```python
from build123d import *

# Parameters (mm, degrees)
BOSS_EXTRUDE1_DEPTH                        = 7
CUT_EXTRUDE1_REACH                         = 39.696
SKETCH2_R                                  = 4
DIAMETER_HOLE1_D                           = 5.5
CBORE_START                                = 4.5
CBORE_FOR_SOCKET_HEAD_CAP_SCREW1_OUTLINE_R = 4
CBORE_FOR_SOCKET_HEAD_CAP_SCREW1_DEPTH     = 4.5
CBORE_FOR_SOCKET_HEAD_CAP_SCREW1_2_OUTLI_R = 2.25
CBORE_FOR_SOCKET_HEAD_CAP_SCREW1_2_DEPTH   = 4.5
TAPPED_HOLE1_D                             = 3.3
CUT_EXTRUDE2_REACH                         = 39.696
SKETCH9_W                                  = 2
SKETCH9_H                                  = 13
SKETCH10_W                                 = 14
SKETCH10_H                                 = 8
CUT_EXTRUDE3_DEPTH                         = 0.4
FILLET1_R                                  = 1
CHAMFER1_SIZE                              = 1


# Read off the part's stored shape, not the designer's step: CBORE for Socket Head Cap Screw1
with BuildPart() as part:
    # Sketch1 → Boss-Extrude1 (new, symmetric)
    with BuildSketch(Plane.XY):
        Polygon((-21, 0), (21, 0), (21, 6), (9, 6), (9, 28), (-9, 28), (-9, 6), (-21, 6), align=None)
    extrude(amount=BOSS_EXTRUDE1_DEPTH, both=True)

    # Sketch2 → Cut-Extrude1 (cut, up to next)
    with BuildSketch(Plane.XY.offset(7), mode=Mode.PRIVATE) as cut_extrude1_sk1:
        with Locations((0, 15)):
            Circle(SKETCH2_R)
    cut_extrude1_tool1 = extrude(cut_extrude1_sk1.sketch, amount=-CUT_EXTRUDE1_REACH, mode=Mode.PRIVATE) & part.part
    add(cut_extrude1_tool1.solids().sort_by_distance((0, 15, 7))[0], mode=Mode.SUBTRACT)

    # Diameter Hole1 (through all)
    with Locations(Plane(origin=(0, 6, 0), x_dir=(1, 0, 0), z_dir=(0, 1, 0))):
        with Locations((-16, 0), (16, 0)):
            Hole(DIAMETER_HOLE1_D / 2)

    # CBORE for Socket Head Cap Screw1 outline → CBORE for Socket Head Cap Screw1 (cut)
    with BuildSketch(Plane.YZ.offset(CBORE_START)):
        with Locations((22.8, 0)):
            Circle(CBORE_FOR_SOCKET_HEAD_CAP_SCREW1_OUTLINE_R)
    extrude(amount=CBORE_FOR_SOCKET_HEAD_CAP_SCREW1_DEPTH, mode=Mode.SUBTRACT)

    # CBORE for Socket Head Cap Screw1 2 outli → CBORE for Socket Head Cap Screw1 2 (cut)
    with BuildSketch(Plane.YZ):
        with Locations((22.8, 0)):
            Circle(CBORE_FOR_SOCKET_HEAD_CAP_SCREW1_2_OUTLI_R)
    extrude(amount=CBORE_FOR_SOCKET_HEAD_CAP_SCREW1_2_DEPTH, mode=Mode.SUBTRACT)

    # Tapped Hole1 (through all)
    with Locations(Plane(origin=(-9, -2.558166827, -1.433608379), x_dir=(0, 0, -1), z_dir=(-1, 0, 0))):
        with Locations((-1.433608379, -25.358166827)):
            Hole(TAPPED_HOLE1_D / 2)

    # Sketch9 → Cut-Extrude2 (cut, up to next)
    with BuildSketch(Plane.XY.offset(7), mode=Mode.PRIVATE) as cut_extrude2_sk1:
        with Locations((0, 21.5)):
            Rectangle(SKETCH9_W, SKETCH9_H)
    cut_extrude2_tool1 = extrude(cut_extrude2_sk1.sketch, amount=-CUT_EXTRUDE2_REACH, mode=Mode.PRIVATE) & part.part
    add(cut_extrude2_tool1.solids().sort_by_distance((0, 21.5, 7))[0], mode=Mode.SUBTRACT)

    # Sketch10 → Cut-Extrude3 (cut)
    with BuildSketch(Plane.XY.offset(7)):
        with Locations((0, 6)):
            Rectangle(SKETCH10_W, SKETCH10_H)
    extrude(amount=-CUT_EXTRUDE3_DEPTH, mode=Mode.SUBTRACT)

    # Fillet1
    fillet1_edges = [part.edges().sort_by_distance(p)[0] for p in [
        (21, 3, 7),
        (-21, 3, -7),
        (15, 6, 7),
        (-21, 6, 0),
        (-9, 6, 0),
        (-9, 28, 0),
        (9, 28, 0),
        (9, 6, 0),
        (21, 6, 0),
        (9, 17, 7),
        (5, 28, 7),
        (-9, 17, 7),
        (-15, 6, 7),
        (-21, 3, 7),
        (-5, 28, -7),
        (-5, 28, 7),
        (-15, 6, -7),
        (-9, 17, -7),
        (5, 28, -7),
        (9, 17, -7),
        (15, 6, -7),
        (21, 3, -7),
    ]]
    fillet(fillet1_edges, radius=FILLET1_R)

    # Chamfer1
    chamfer1_edges = [part.edges().sort_by_distance(p)[0] for p in [
        (0, 11, 7),
        (0, 11, -7),
    ]]
    chamfer(chamfer1_edges, length=CHAMFER1_SIZE - 0.0001)  # a hair under: the kernel refuses the full size


solid = part.part
```
Geometry check sheet. Reference: the model listing, model coordinates, mm. A direction names the side the tool comes from. Round coordinates to 2 decimals unless told otherwise and drop trailing zeros. Order: outer loops, then holes, each group sorted by start corner. A loop starts at its lowest first (then second) coordinate and runs counter-clockwise, first axis right, second up. Notation, with made-up numbers: (80.25, -28) - (113.25, -28) arc R18 ccw to (113.25, -17) - close; hole circle Ø7 at (86.25, 75.5). An arc over 180 degrees is marked (long way). Use a Markdown table: item, result. Add a question column.
1) Section check C-C (y = 15). Record the cut outline in (x, z), then the cut area to 3 significant figures.
2) Thickness scan on line 1 along Z through (x, y) = (3.1, 22.8); line 2 along Z through (x, y) = (-5.5, 22.8); line 3 along X through (y, z) = (26.25, 3). Record the ranges inside material, lowest first.
3) Section check D-D (x = -15.5). Record the cut outline in (y, z), then the cut area to 3 significant figures.
4) Set-up check for faces 4 (the flat face through (13, 6, 0)), 5 (the cylindrical face through (14.93, 5.699, 6.715)), 6 (the cylindrical face through (-8.699, 16.86, 6.715)), 7 (the cylindrical face through (2.726, 20.552, 0.099)), 8 (the conical face through (-0.171, 10.844, -6.16)): record each of +Z, -Z, +X, -X, +Y, -Y from which the full face is reachable in a straight line by a thin tool's end or side.
5) Mould release check, pull along Y, two halves, no side actions. Record for faces 1 (the cylindrical face through (6.719, 26.495, -1.532)), 2 (the cylindrical face through (8.715, 27.699, 0.084)), 3 (the cylindrical face through (-20.715, 2.465, 6.699)): released by +Y, released by -Y, zero draft, split by the parting line, or undercut.
6) Section check A-A (y = 22.8). Record the cut outline in (x, z), then the cut area to 3 significant figures.
7) Gauge pin test, flat ends, axial feed: P1, Ø7, axis at x = 0, y = 15, coming from the +Z side; P2, Ø6, axis at y = 13.5, z = -1.5, coming from the -X side; P3, Ø3, axis at x = 14, z = -1.5, coming from the +Y side; P4, Ø3.5, axis at y = 12.5, z = -2.5, coming from the +X side. Record the tip position at first contact, or that the pin passes through.
Established:
| question | item | result |
|---|---|---|
| 1 | outline | (-9, -6) arc R1 ccw to (-8, -7) - (-5, -7) - (-4, -6) - (-4, 6) - (-5, 7) - (-8, 7) arc R1 ccw to (-9, 6) - close; (4, -6) - (5, -7) - (8, -7) arc R1 ccw to (9, -6) - (9, 6) arc R1 ccw to (8, 7) - (5, 7) - (4, 6) - close |
| 1 | area | 137 mm2 |
| 2 | line 1 | -7 to -2.25, 2.25 to 7 |
| 2 | line 2 | -7 to -1.65, 1.65 to 7 |
| 2 | line 3 | -9 to -1, 1 to 9 |
| 3 | outline | (0, -7) - (5, -7) arc R1 ccw to (6, -6) - (6, -2.7) - (0, -2.7) - close; (0, 2.7) - (6, 2.7) - (6, 6) arc R1 ccw to (5, 7) - (0, 7) - close |
| 3 | area | 51.1 mm2 |
| 4 | face 4 | +Z, -Z, +X, +Y |
| 4 | face 5 | +Z, +X, +Y |
| 4 | face 6 | +Z, -X, +Y |
| 4 | face 7 | +X |
| 4 | face 8 | -Z |
| 5 | face 1 | undercut |
| 5 | face 2 | released by +Y |
| 5 | face 3 | zero draft |
| 6 | outline | (-9, -6) arc R1 ccw to (-8, -7) - (-1, -7) - (-1, -1.65) - (-9, -1.65) - close; (-9, 1.65) - (-1, 1.65) - (-1, 7) - (-8, 7) arc R1 ccw to (-9, 6) - close; (1, -7) - (8, -7) arc R1 ccw to (9, -6) - (9, -4) - (4.5, -4) - (4.5, -2.25) - (1, -2.25) - close; (1, 2.25) - (4.5, 2.25) - (4.5, 4) - (9, 4) - (9, 6) arc R1 ccw to (8, 7) - (1, 7) - close |
| 6 | area | 145 mm2 |
| 7 | P1 | through |
| 7 | P2 | x = -9 |
| 7 | P3 | y = 6 |
| 7 | P4 | x = 9 |
